Check sheet for the modelled part. Datum: model origin and axes. Units: mm. Face numbers are marked on the shaded views. A direction names the side the tool comes from. Round coordinates to 2 decimals unless told otherwise and drop trailing zeros. Order: outer loops, then holes, each group sorted by start corner. A loop starts at its lowest first (then second) coordinate and runs counter-clockwise, first axis right, second up.
(1) Sectioned sample at A-A, the plane x = 0. Enter the section's corners in (y, z).
(2) Thickness scan on probe 1 along X at (y, z) = (-16, 24); probe 2 along Y at (x, z) = (-17, 17.5); probe 3 along X at (y, z) = (19.5, 39.5). Record the ranges inside material, lowest first.
(3) Sectioned sample at D-D, the plane x = 50. Enter the section's corners in (y, z).
(4) Sectioned sample at B-B, the plane y = -12.5. Enter the section's corners in (x, z), and give its area (3 significant figures).
(5) Sectioned sample at C-C, the plane y = 22. Enter the section's corners in (x, z).
(6) Tool access check on the marked faces 1 and 2. Record the directions out of +Z, -Z, +X, -X, +Y, -Y that give a thin tool (end or side, any length) a straight path to the whole face; none if there is none.
(7) Depth check by flat-ended pin: pin 1 (3 mm diameter, centred on x = -47, y = -14, fed in from +Z). Enter the tip coordinate at first touch or a pass-through.
(8) Mould release check, pull along X, two halves, no side actions. Record for the marked faces 3, 4 and 5: released by +X, released by -X, zero draft, split by the parting line, or undercut.
```python
from build123d import *

# Parameters (mm, degrees)
SKETCH1_W           = 120
SKETCH1_H           = 80
BOSS_EXTRUDE1_DEPTH = 50
SKETCH3_R           = 5
BOSS_EXTRUDE2_DEPTH = 10


with BuildPart() as part:
    # Sketch1 → Boss-Extrude1 (new body)
    with BuildSketch(Plane.XY):
        Rectangle(SKETCH1_W, SKETCH1_H)
    extrude(amount=BOSS_EXTRUDE1_DEPTH)

    # Sketch3 → Boss-Extrude2 (add)
    with BuildSketch(Plane.XY.offset(50)):
        with Locations((50, 25)):
            Circle(SKETCH3_R)
        with Locations((-50, -25)):
            Circle(SKETCH3_R)
    extrude(amount=BOSS_EXTRUDE2_DEPTH)

    # Sketch2 → Cut-Revolve2 (revolve, cut)
    with BuildSketch(Plane.XY.offset(50)):
        with BuildLine():
            Line((-35, 40), (-35, 25))
            Line((-35, 25), (-46.913025467, 5.144957554))
            ThreePointArc((-46.913025467, 5.144957554), (-48.33809621, 0), (-46.913025467, -5.144957554))
            Line((-46.913025467, -5.144957554), (-35, -25))
            Line((-35, -25), (-35, -40))
            Line((-35, -40), (0, -40))
            Line((0, -40), (0, 40))
            Line((0, 40), (-35, 40))
        make_face()
    revolve(axis=Axis((0, 43.927138889, 50), (0, -1, 0)), mode=Mode.SUBTRACT)


solid = part.part
```
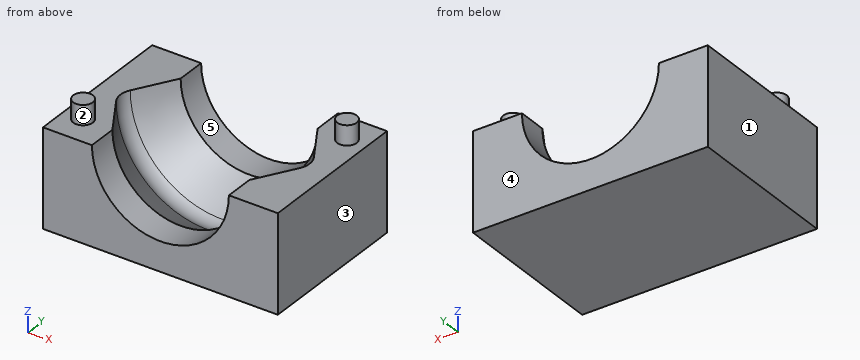
Derived:
1. outline: (-40, 0) - (40, 0) - (40, 15) - (25, 15) - (5.14, 3.09) arc R10 cw to (-5.14, 3.09) - (-25, 15) - (-40, 15) - close
2. probe 1: x = -60 to -30.92, 30.92 to 60
2. probe 2: y = -40 to -22.2, 22.2 to 40
2. probe 3: x = -60 to -36.83, 36.83 to 60
3. outline: (-40, 0) - (40, 0) - (40, 50) - (30, 50) - (30, 60) - (20, 60) - (20, 50) - (-40, 50) - close
4. outline: (-60, 0) - (60, 0) - (60, 50) - (42.5, 50) arc R42.5 cw to (-42.5, 50) - (-60, 50) - close
4. area: 3,160 mm2
5. outline: (-60, 0) - (60, 0) - (60, 50) - (54, 50) - (54, 60) - (46, 60) - (46, 50) - (36.8, 50) arc R36.8 cw to (-36.8, 50) - (-60, 50) - close
6. face 1: +Z, -Z, -X, +Y, -Y
6. face 2: +Z
7. pin 1: stops at z = 50
8. face 3: released by +X
8. face 4: zero draft
8. face 5: undercut
